Input: part model. Units: mm. Frame: model coordinates. A direction names the side the tool comes from. Give positions to 0.01 mm unless a question says otherwise; leave off trailing zeros. Order: outer loops, then holes, each group sorted by start corner. A loop starts at its lowest first (then second) coordinate and runs counter-clockwise, first axis right, second up.
```python
from build123d import *

# Parameters (mm, degrees)
F0_W     = 63.5
F0_H     = 88.9
F1_DEPTH = 12.192
F2_D     = 9.906
F6_DEPTH = 44.45
F7_R     = 12.7


# Not quite as in the source:
# - a pattern or mirror of a feature is missing from the dataset's text; its kind, count and spacing are read off the source's solid


with BuildPart() as f1:
    # F0 (on Top) → F1 (new body)
    with BuildSketch(Plane.XY):
        Rectangle(F0_W, F0_H)
    extrude(amount=-F1_DEPTH)

    # F2 (through all)
    with Locations(Plane.XY):
        with Locations((19.05, -31.75)):
            f2 = Hole(F2_D / 2)

    # F2_copies: F2 across plane
    add(f2.mirror(Plane(origin=(0, 0, 0), x_dir=(0.8574929257, 0.5144957554, 0), z_dir=(-0.5144957554, 0.8574929257, 0))), mode=Mode.SUBTRACT)

    # F2_copies1: F2 across plane
    add(f2.mirror(Plane(origin=(0, 0, 0), x_dir=(0, 0, -1), z_dir=(-1, 0, 0))), mode=Mode.SUBTRACT)

    # F2_copies2: F2 across plane
    add(f2.mirror(Plane.ZX), mode=Mode.SUBTRACT)

    # F5 (on line) → F6 (join, through all)
    with BuildSketch(Plane(origin=(11.1553204089, -19.3215817229, 0), x_dir=(0.8660254038, 0.5, 0), z_dir=(0.5, -0.8660254038, 0))):
        Polygon((-16.4748365541, 33.782), (-16.4748365541, 0), (15.2751634459, 0), (15.2751634459, 33.782), (11.9731634459, 33.782), (2.5751634459, 19.0759231813), (2.5751634459, 14.732), (-3.7748365541, 14.732), (-3.7748365541, 19.0759231813), (-13.1728365541, 33.782), align=None)
    extrude(amount=-F6_DEPTH)

    # F7
    f7_edges = [f1.edges().sort_by_distance(p)[0] for p in [
        (31.75, -44.45, -6.096),
        (31.75, 44.45, -6.096),
        (-31.75, 44.45, -6.096),
        (-31.75, -44.45, -6.096),
    ]]
    fillet(f7_edges, radius=F7_R)


solid = f1.part
```
1) Line query: probe 1 along Y at (x, z) = (-19, -3); probe 2 along X at (y, z) = (33.5, -5); probe 3 along Z at (x, y) = (-21.5, 22.5). Output: solid intervals per line, ascending.
2) Cut plane C-C (x = 23). Return the cut outline in (y, z).
3) Reachability of faces 1 (the face through (-14.07, -8.58, 17.13)), 2 (the face through (0, -1, 14.732)), 3 (the face through (-11.782, 18.762, 13.374)) from +Z, -Z, +X, -X, +Y, -Y: full face, straight path, thin tool, end or side. Return the list, or none.
4) First-contact query: P1, Ø6, axis at x = -20, y = -30.5, coming from the -Z side; P2, Ø13, axis at x = 19.05, y = 31.75, coming from the +Z side; P3, Ø6, axis at x = 5.5, z = 24, coming from the -Y side; P4, Ø5, axis at x = 2.5, z = 5.5, coming from the -Y side. Flat tips, straight axial feed; report the tip coordinate or a pass-through.
5) Cut plane B-B (z = -2.5). Return the cut outline in (x, y), then the cut area to 3 significant figures.
6) Cut plane D-D (y = -15.5). Return the cut outline in (x, z).
7) Cut plane A-A (z = 18). Return the cut outline in (x, y).
Geometry says:
1. probe 1: y = -44.45 to -36.7, -26.8 to 26.8, 36.7 to 44.45
1. probe 2: x = -31.63 to -23.68, -14.42 to 14.42, 23.68 to 31.63
1. probe 3: z = -12.19 to 0
2. outline: (-43.82, -12.19) - (-34.74, -12.19) - (-34.74, 0) - (-43.82, 0) - close; (-28.76, -12.19) - (28.76, -12.19) - (28.76, 0) - (-9.29, 0) - (-9.29, 33.78) - (-12.48, 33.78) - (-12.48, 0) - (-28.76, 0) - close; (34.74, -12.19) - (43.82, -12.19) - (43.82, 0) - (34.74, 0) - close
3. face 1: +Z, -X, -Y
3. face 2: +Z
3. face 3: +Z, -X, +Y
4. P1: passes through
4. P2: stops at z = 0
4. P3: stops at y = -24.32
4. P4: stops at y = -25.76
5. outline: (-31.75, -31.75) arc R12.7 ccw to (-19.05, -44.45) - (19.05, -44.45) arc R12.7 ccw to (31.75, -31.75) - (31.75, 31.75) arc R12.7 ccw to (19.05, 44.45) - (-19.05, 44.45) arc R12.7 ccw to (-31.75, 31.75) - close; hole circle Ø9.91 at (-19.05, -31.75); hole circle Ø9.91 at (-19.05, 31.75); hole circle Ø9.91 at (19.05, -31.75); hole circle Ø9.91 at (19.05, 31.75)
5. area: 5,200 mm2
6. outline: (-31.75, -12.19) - (31.75, -12.19) - (31.75, 0) - (17.77, 0) - (17.77, 27.01) - (11.92, 19.08) - (11.92, 14.73) - (4.59, 14.73) - (4.59, 19.08) - (-6.26, 33.78) - (-10.07, 33.78) - (-10.07, 0) - (-31.75, 0) - close
7. outline: (-25.34, 10.94) - (-3.11, -27.56) - (7.89, -21.21) - (-14.34, 17.29) - close; (-8.84, 20.46) - (13.39, -18.03) - (24.38, -11.68) - (2.16, 26.81) - close
